from build123d import *

# Parameters (mm, degrees)
BOSS_EXTRUDE1_DEPTH     = 1.5875
BOSS_EXTRUDE2_START     = 1.5875
SKETCH4_R               = 1
BOSS_EXTRUDE2_DEPTH     = 6.35
CUT_EXTRUDE1_DEPTH      = 212.336707427
CUT_EXTRUDE1_DEPTH_BACK = 212.336707427


with BuildPart() as part:
    # Sketch2 → Boss-Extrude1 (new, symmetric)
    with BuildSketch(Plane.XY):
        Polygon((46.2, -46.2), (0, -46.2), (0, -106.2), (46.2, -106.2), (46.2, -146.2), (106.2, -146.2), (106.2, -106.2), (152.4, -106.2), (152.4, -46.2), (106.2, -46.2), (106.2, -6.2), (46.2, -6.2), align=None)
    extrude(amount=BOSS_EXTRUDE1_DEPTH, both=True)

    # Sketch4 → Boss-Extrude2 (add)
    with BuildSketch(Plane.XY.offset(BOSS_EXTRUDE2_START)):
        with Locations((53.34, -11.2)):
            Circle(SKETCH4_R)
        with Locations((68.58, -11.2)):
            Circle(SKETCH4_R)
        with Locations((99.06, -11.2)):
            Circle(SKETCH4_R)
        with Locations((83.82, -11.2)):
            Circle(SKETCH4_R)
        with Locations((99.06, -24.533333333)):
            Circle(SKETCH4_R)
        with Locations((99.06, -37.866666667)):
            Circle(SKETCH4_R)
        with Locations((114.3, -51.2)):
            Circle(SKETCH4_R)
        with Locations((99.06, -51.2)):
            Circle(SKETCH4_R)
        with Locations((144.78, -51.2)):
            Circle(SKETCH4_R)
        with Locations((129.54, -51.2)):
            Circle(SKETCH4_R)
        with Locations((144.78, -61.2)):
            Circle(SKETCH4_R)
        with Locations((144.78, -71.2)):
            Circle(SKETCH4_R)
        with Locations((144.78, -81.2)):
            Circle(SKETCH4_R)
        with Locations((144.78, -91.2)):
            Circle(SKETCH4_R)
        with Locations((144.78, -101.2)):
            Circle(SKETCH4_R)
        with Locations((114.3, -101.2)):
            Circle(SKETCH4_R)
        with Locations((129.54, -101.2)):
            Circle(SKETCH4_R)
        with Locations((99.06, -101.2)):
            Circle(SKETCH4_R)
        with Locations((99.06, -114.533333333)):
            Circle(SKETCH4_R)
        with Locations((99.06, -127.866666667)):
            Circle(SKETCH4_R)
        with Locations((99.06, -141.2)):
            Circle(SKETCH4_R)
        with Locations((83.82, -141.2)):
            Circle(SKETCH4_R)
        with Locations((68.58, -141.2)):
            Circle(SKETCH4_R)
        with Locations((53.34, -141.2)):
            Circle(SKETCH4_R)
        with Locations((53.34, -127.866666667)):
            Circle(SKETCH4_R)
        with Locations((53.34, -114.533333333)):
            Circle(SKETCH4_R)
        with Locations((53.34, -101.2)):
            Circle(SKETCH4_R)
        with Locations((38.1, -101.2)):
            Circle(SKETCH4_R)
        with Locations((7.62, -101.2)):
            Circle(SKETCH4_R)
        with Locations((22.86, -101.2)):
            Circle(SKETCH4_R)
        with Locations((7.62, -91.2)):
            Circle(SKETCH4_R)
        with Locations((7.62, -81.2)):
            Circle(SKETCH4_R)
        with Locations((7.62, -71.2)):
            Circle(SKETCH4_R)
        with Locations((7.62, -51.2)):
            Circle(SKETCH4_R)
        with Locations((7.62, -61.2)):
            Circle(SKETCH4_R)
        with Locations((22.86, -51.2)):
            Circle(SKETCH4_R)
        with Locations((53.34, -51.2)):
            Circle(SKETCH4_R)
        with Locations((38.1, -51.2)):
            Circle(SKETCH4_R)
        with Locations((53.34, -37.866666667)):
            Circle(SKETCH4_R)
        with Locations((53.34, -24.533333333)):
            Circle(SKETCH4_R)
    extrude(amount=BOSS_EXTRUDE2_DEPTH)

    # Sketch3 → Cut-Extrude1 (cut, two sides: drawn at the far end of the back side and taken through both)
    with BuildSketch(Plane.XY.offset(-CUT_EXTRUDE1_DEPTH_BACK)):
        with BuildLine():
            Line((18.425, -76.2), (18.425, -109.794189798))
            ThreePointArc((18.425, -109.794189798), (16.7, -111.519189798), (14.975, -109.794189798))
            Line((14.975, -109.794189798), (14.975, -76.2))
            ThreePointArc((14.975, -76.2), (16.7, -74.475), (18.425, -76.2))
        make_face()
        with BuildLine():
            Line((96.2632, -57.8618), (96.2632, -157.352229572))
            ThreePointArc((96.2632, -157.352229572), (94.5382, -159.077229572), (92.8132, -157.352229572))
            Line((92.8132, -157.352229572), (92.8132, -57.8618))
            ThreePointArc((92.8132, -57.8618), (94.5382, -56.1368), (96.2632, -57.8618))
        make_face()
    extrude(amount=CUT_EXTRUDE1_DEPTH + CUT_EXTRUDE1_DEPTH_BACK, mode=Mode.SUBTRACT)


solid = part.part
Build history of the part. All positions in model axes, mm. A direction names the side the tool comes from. Coordinates: 2 decimals unless noted, no trailing zeros. Order: outer loops, then holes, each group sorted by start corner. A loop starts at its lowest first (then second) coordinate and runs counter-clockwise, first axis right, second up. Notation, with made-up numbers: (63.5, -27) - (87.5, -27) arc R18 ccw to (87.5, -7) - close; hole circle Ø8 at (19.5, 73.5). An arc over 180 degrees is marked (long way). Write item = value, one per line. Start each with the question number.
1) Saw through at B-B on z = 0. Write the cut outline in (x, y) (3 decimals), then the cut area to 3 significant figures.
2) Saw through at C-C on y = -42. Write the cut outline in (x, z), then the cut area to 4 significant figures.
3) Wall check: line 1 along X through (y, z) = (-62.5, -0.75); line 2 along Z through (x, y) = (119, -66); line 3 along X through (y, z) = (-37, -0.5). Give the ranges that are in metal, low to high. Write a range as from..to.
4) Flat gauge pins, fed straight in: pin 1 Ø3.5 at (x, z) = (134, 0) entering from +Y; pin 2 Ø12 at (x, y) = (66.5, -94) entering from +Z; pin 3 Ø1.6 at (y, z) = (-123, -0.5) entering from -X. Where does each tip first touch, or does it go through?
5) Two-plate mould, pull along X, no slides. Class faces 1 (the face through (32, -106.2, 0)), 2 (the face through (96.263, -101, 0)), 3 (the face through (94.5, -56.137, -0.022)), 4 (the face through (0, -76, 0)): pulls with the +X half, pulls with the -X half, needs draft (parallel to the pull), parting line crosses it, or undercut.
6) 3-axis set-ups, long thin cutter, end or side, ignore diameter. For faces 5 (the face through (7, -106.2, 0)), 6 (the face through (130, -46.2, 0)), 7 (the face through (46.2, -26, 0)): which of +Z, -Z, +X, -X, +Y, -Y reach the whole face in a straight line?
7) Saw through at A-A on y = -124. Write the cut outline in (x, z), then the cut area to 3 significant figures.
8) Saw through at D-D on x = 74.5. Write the cut outline in (y, z), then the cut area to 4 significant figures.
From the geometry:
q1.outline = (0, -106.2) - (14.975, -106.2) - (14.975, -76.2) arc R1.725 cw to (18.425, -76.2) - (18.425, -106.2) - (46.2, -106.2) - (46.2, -146.2) - (92.813, -146.2) - (92.813, -57.862) arc R1.725 cw to (96.263, -57.862) - (96.263, -146.2) - (106.2, -146.2) - (106.2, -106.2) - (152.4, -106.2) - (152.4, -46.2) - (106.2, -46.2) - (106.2, -6.2) - (46.2, -6.2) - (46.2, -46.2) - (0, -46.2) - close
q1.area = 13,500 mm^2
q2.outline = (46.2, -1.59) - (106.2, -1.59) - (106.2, 1.59) - (46.2, 1.59) - close
q2.area = 190.5 mm^2
q3.line_1 = 0..92.81, 96.26..152.4
q3.line_2 = -1.59..1.59
q3.line_3 = 46.2..106.2
q4.pin_1 = -46.2
q4.pin_2 = 1.59
q4.pin_3 = 46.2
q5.face_1 = needs draft
q5.face_2 = undercut
q5.face_3 = undercut
q5.face_4 = pulls with the -X half
q6.face_5 = +Z, -Z, -X, -Y
q6.face_6 = +Z, -Z, +X, +Y
q6.face_7 = +Z, -Z, -X, +Y
q7.outline = (46.2, -1.59) - (92.81, -1.59) - (92.81, 1.59) - (46.2, 1.59) - close; (96.26, -1.59) - (106.2, -1.59) - (106.2, 1.59) - (96.26, 1.59) - close
q7.area = 180 mm^2
q8.outline = (-146.2, -1.59) - (-6.2, -1.59) - (-6.2, 1.59) - (-146.2, 1.59) - close
q8.area = 444.5 mm^2
